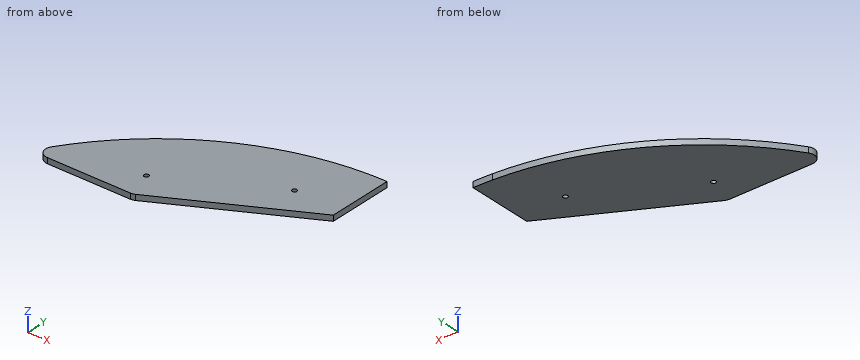
Autodesk Inventor part; units mm, degrees
ref_plane "YZ Plane" through (0, 0, 0) normal (1, 0, 0) x (0, 1, 0)
ref_plane "XZ Plane" through (0, 0, 0) normal (0, 1, 0) x (-1, 0, 0)
ref_plane "XY Plane" through (0, 0, 0) normal (0, 0, 1) x (1, 0, 0)
sketch "Sketch1" plane through (0, 0, 0) normal (0, 0, 1) x (1, 0, 0)
  circle A0 centre (0, 0) radius 300
  dimension "d0" = 600
extrude "Extrusion1" add sketch "Sketch1" along normal blind 6
sketch "Sketch2" plane through (0, 0, 6) normal (0, 0, 1) x (1, 0, 0)
  line L0 (-170, -250) -> (170, -250)
  line L1 (170, -250) -> (170, 250)
  line L2 (170, 250) -> (-170, 250)
  line L3 (-170, 250) -> (-170, -250)
  line L4 (-170, -250) -> (170, 250) construction
  line L5 (170, -250) -> (-170, 250) construction
  line L6 (-150, 230) -> (150, 230)
  line L7 (150, 230) -> (150, -230)
  line L8 (150, -230) -> (-150, -230)
  line L9 (-150, -230) -> (-150, 230)
  point P0 (0, 0)
  dimension "d3" = 340
  dimension "d4" = 500
  dimension "d5" = 20
sketch "Sketch3" plane through (0, 0, 6) normal (0, 0, 1) x (1, 0, 0)
  line L0 (0, 0) -> (-261.0308, 150.7062)
  line L1 (0, 0) -> (261.1835, 150.7944)
  line L2 (0, 0) -> (299.5929, 0) construction
  arc A0 (261.1835, 150.7944) -> (-261.0308, 150.7062) centre (0.1023, -3.0238) ccw
  dimension "d6" = 120
  dimension "d7" = 30
extrude "Extrusion2" cut sketch "Sketch3" along normal through all both and the other way through all keep common part
sketch "Sketch4" plane through (0, 0, 6) normal (0, 0, 1) x (1, 0, 0)
  arc A0 (-20.2802, 299.3137) -> (-259.8076, 150) centre (0, 0) ccw
  line L0 (259.8076, 150) -> (0, 0)
  line L1 (-259.8076, 150) -> (259.8076, 150)
  line L2 (259.8076, 150) -> (0, 0)
  line L3 (0, 0) -> (-259.8076, 150)
extrude "Extrusion3" cut sketch "Sketch4" against normal through all
sketch "Sketch5" plane through (0, 0, 6) normal (0, 0, 1) x (1, 0, 0)
  line L0 (-259.8076, 150) -> (259.8076, 150)
  arc A0 (259.8076, 150) -> (0, 300) centre (0, 0) ccw
  arc A1 (0, 300) -> (-20.2802, 299.3137) centre (0.1023, -3.0238) ccw
  arc A2 (-20.2802, 299.3137) -> (-259.8076, 150) centre (0, 0) ccw
  line L1 (-150, 230) -> (150, 230)
  line L2 (-150, -230) -> (-150, 230)
  line L3 (170, 250) -> (-170, 250)
  line L4 (-170, 250) -> (-170, -250)
  line L5 (-259.8076, 150) -> (259.8076, 150)
  line L6 (-150, 150) -> (0, 230)
  line L7 (0, 300) -> (0, 230)
extrude "Extrusion4" cut sketch "Sketch5" against normal through all contours L6 L7 L3 A0 L0 | L3 L7 A0
fillet "Fillet1" radius 10 2 edges at (-259.8076, 150, 3) (-150, 150, 3)
sketch "Sketch6" plane through (0, 0, 6) normal (0, 0, 1) x (1, 0, 0)
  line L0 (0, 230) -> (0, 300)
  line L1 (170, 250) -> (-170, 250)
  line L2 (-170, 250) -> (-170, -250)
  point P0 (0, 0)
  point P1 (-160, 180)
  point P2 (-50, 240)
  dimension "d15" = 50
  dimension "d16" = 70
  dimension "d17" = 10
  dimension "d18" = 10
hole "Hole1" at (-160, 180, 6) at (-50, 240, 6) direction (0, 0, -1) diameter 5 end through all
properties part number "beltMount"
Geometry check sheet. Reference: the model listing, model coordinates, mm. Give positions to 0.01 mm unless a question says otherwise; leave off trailing zeros. Order: outer loops, then holes, each group sorted by start corner. A loop starts at its lowest first (then second) coordinate and runs counter-clockwise, first axis right, second up. Notation, with made-up numbers: (-11.75, 39.5) - (-0.75, 39.5) arc R21 cw to (-0.75, 70.5) - close; hole circle Ø8 at (48, -19). An arc over 180 degrees is marked (long way). Use one line per item in the form item = value.
1) Sectioned sample at D-D (y = 283). Record the boundary of the cut face in (x, z), and give its area (3 significant figures).
Working result:
outline = (-99.55, 0) - (0, 0) - (0, 6) - (-99.55, 6) - close
area = 597 mm^2
2) Sectioned sample at B-B (x = -50). Record the boundary of the cut face in (y, z).
Working result:
outline = (203.33, 0) - (237.5, 0) - (237.5, 6) - (203.33, 6) - close; (242.5, 0) - (295.8, 0) - (295.8, 6) - (242.5, 6) - close
3) Sectioned sample at A-A (y = 240). Record the boundary of the cut face in (x, z).
Working result:
outline = (-180, 0) - (-52.5, 0) - (-52.5, 6) - (-180, 6) - close; (-47.5, 0) - (0, 0) - (0, 6) - (-47.5, 6) - close
4) Depth check by flat-ended pin: pin 1 Ø1 at (y, z) = (197, 0.5) entering from +X; pin 2 Ø1 at (x, z) = (-208.5, 4) entering from +Y. Enter the tip coordinate at first touch or a pass-through.
Working result:
pin_1 = -60.94
pin_2 = 216.19
5) Material ranges on probe 1 along Y at (x, z) = (-160, 2.25); probe 2 along X at (y, z) = (180, 1.8); probe 3 along Y at (x, z) = (-50, 3.4), recorded low to high. Write a range as from..to.
Working result:
probe_1 = 150..177.5, 182.5..253.77
probe_2 = -240..-162.5, -157.5..-93.75
probe_3 = 203.33..237.5, 242.5..295.8
6) Sectioned sample at C-C (z = 3.85). Record the boundary of the cut face in (x, y), and give its area (3 significant figures).
Working result:
outline = (-250.21, 165.52) arc R10 ccw to (-241.87, 150) - (-152.5, 150) arc R10 ccw to (-147.79, 151.18) - (0, 230) - (0, 300) arc R303.02 ccw to (-20.29, 299.31) arc R300 ccw to start; hole circle Ø5 at (-160, 180); hole circle Ø5 at (-50, 240)
area = 21,500 mm^2
